```python
from build123d import *

# Parameters (mm, degrees)
F0_R           = 32.5
F1_DEPTH       = 80
F2_R           = 37.5
F3_DEPTH       = 13
F4_R           = 37.5
F5_DEPTH       = 17
F6_R           = 2
F8_D           = 6.6
F8_CBORE_D     = 11.25
F8_CBORE_DEPTH = 14
F9_R           = 1


with BuildPart() as f1:
    # F0 (on Front) → F1 (new body)
    with BuildSketch(Plane.XZ):
        Circle(F0_R)
    extrude(amount=F1_DEPTH)

    # F2 (on Front) → F3 (join)
    with BuildSketch(Plane.XZ):
        Circle(F2_R)
    extrude(amount=-F3_DEPTH)

    # F4 (on face) → F5 (join)
    with BuildSketch(Plane.XZ.offset(80)):
        Circle(F4_R)
    extrude(amount=F5_DEPTH)

    # F6
    f6_edges = [f1.edges().sort_by_distance(p)[0] for p in [
        (-32.5, 0, 0),
        (-37.5, -97, 0),
        (-32.5, -80, 0),
    ]]
    fillet(f6_edges, radius=F6_R)

    # F8 (through all)
    with Locations(Plane.XZ.offset(97)):
        with Locations((0, 12.5), (0, -12.5)):
            CounterBoreHole(F8_D / 2, F8_CBORE_D / 2, F8_CBORE_DEPTH)

    # F9
    f9_edges = [f1.edges().sort_by_distance(p)[0] for p in [
        (-37.5, 0, 0),
        (-37.5, -80, 0),
    ]]
    fillet(f9_edges, radius=F9_R)


solid = f1.part
```
The listing builds one solid part. Answer for the finished solid, in the listing's coordinates (mm). A direction names the side the tool comes from. Give positions to 0.01 mm unless a question says otherwise; leave off trailing zeros. Order: outer loops, then holes, each group sorted by start corner. A loop starts at its lowest first (then second) coordinate and runs counter-clockwise, first axis right, second up. Notation, with made-up numbers: (36, 74.5) -> (70, 74.5) arc R23 cw to (70, 85.5) -> close; hole circle Ø7 at (-21, -0.5). An arc over 180 degrees is marked (long way). Answer as a JSON object with one key per item and string values. Group by question number.
Item 1: Determine the mould class of faces 4 (the flat face through (27, 0, 22)), 5 (the flat face through (27, -80, 22)), 6 (the cylindrical face through (0.72, -34.33, -15.72)), 7 (the flat face through (-1, 13, 1)) for opening direction Y: pulls with the +Y half, pulls with the -Y half, needs draft (parallel to the pull), parting line crosses it, or undercut.
Item 2: The part is cut by section A-A on y = -54. Write down the section's boundary in (x, z).
Item 3: A tool of negligible diameter and unlimited length cuts with its end or side. For faces 1 (the flat face through (4, -83, 13)), 2 (the cylindrical face through (31, -39.47, 9.76)), 3 (the cylindrical face through (0.72, -34.33, 9.28)), from which of +Z, -Z, +X, -X, +Y, -Y can it reach the whole face along a straight path? Write none if from no direction.
Item 4: The part is cut by section B-B on x = 0. Give the number of separate pieces and of enclosed holes in the cut face, and give its area (3 significant figures).
Item 5: Consider L1, parallel to Z at x = 0, y = -92 (3 decimals); L2, parallel to Z at x = 0, y = -57; L3, parallel to X at y = -90, z = -12. Determine where each line is inside the solid, lowest interval first. Write a range as from..to.
Item 6: Flat-ended cylindrical pins translate along their axes: pin 1 (5.5 mm diameter, centred on x = 0, z = -12.5, fed in from -Y); pin 2 (1.5 mm diameter, centred on x = 28.5, y = -80, fed in from -Z); pin 3 (1 mm diameter, centred on x = 27, y = -54.5, fed in from -Z); pin 4 (9 mm diameter, centred on x = 3, z = -12.5, fed in from -Y). Find the tip coordinate at first contact, or state that the pin passes through.
Result set:
{
 "1": {"face 4": "undercut", "face 5": "undercut", "face 6": "needs draft", "face 7": "pulls with the +Y half"},
 "2": {"outline": "circle Ø65 at (0, 0); hole circle Ø6.6 at (0, -12.5); hole circle Ø6.6 at (0, 12.5)"},
 "3": {"face 1": "-Y", "face 2": "none", "face 3": "+Y, -Y"},
 "4": {"separate pieces": "3", "enclosed holes": "0", "area": "5,870 mm²"},
 "5": {"L1": "-37.5..-18.125, -6.875..6.875, 18.125..37.5", "L2": "-32.5..-15.8, -9.2..9.2, 15.8..32.5", "L3": "-35.53..-5.6, 5.6..35.53"},
 "6": {"pin 1": "through", "pin 2": "z = -24.81", "pin 3": "z = -18.81", "pin 4": "y = -97"}
}
